Geometry: final body of the model. Coordinates: model frame, mm. Give positions to 0.01 mm unless a question says otherwise; leave off trailing zeros. Order: outer loops, then holes, each group sorted by start corner. A loop starts at its lowest first (then second) coordinate and runs counter-clockwise, first axis right, second up. Notation, with made-up numbers: (36, 10.5) - (92, 10.5) arc R30 cw to (92, 40.5) - close; hole circle Ø11 at (-19.5, 88.25). An arc over 180 degrees is marked (long way). One line per question, with ' | ' between items. Start each with the question number.
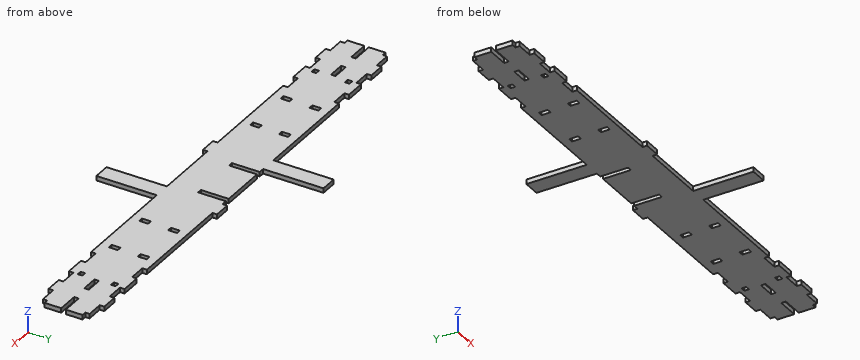
from build123d import *

# Parameters (mm, degrees)
SKETCH1_W           = 4.1
SKETCH1_H           = 4.1
SKETCH1_H_2         = 8
SKETCH1_W_2         = 15
BOSS_EXTRUDE1_DEPTH = 4.1
SKETCH2_W           = 15
SKETCH2_H           = 4.1
TOP_RIGHT_DEPTH     = 50.1
SKETCH3_W           = 15
SKETCH3_H           = 4.1
BOTTOM_LEFT_DEPTH   = 50.1


with BuildPart() as part:
    # Sketch1 → Boss-Extrude1 (new body)
    with BuildSketch(Plane.XY):
        Polygon((-205, -20.9), (-205, -25), (-190, -25), (-190, -20.9), (-175, -20.9), (-175, -25), (-157, -25), (-157, -20.9), (-142, -20.9), (-142, -25), (-45, -25), (-45, -79.2), (-30, -79.2), (-30, -25), (30, -25), (30, -79.2), (45, -79.2), (45, -25), (142, -25), (142, -20.9), (157, -20.9), (157, -25), (175, -25), (175, -20.9), (190, -20.9), (190, -25), (205, -25), (205, -20.9), (220, -20.9), (220, -17.05), (224.1, -17.05), (224.1, -2.05), (205, -2.05), (205, 2.05), (224.1, 2.05), (224.1, 17.05), (220, 17.05), (220, 20.9), (205, 20.9), (205, 25), (190, 25), (190, 20.9), (175, 20.9), (175, 25), (157, 25), (157, 20.9), (142, 20.9), (142, 25), (45, 25), (45, 79.2), (30, 79.2), (30, 25), (25, 25), (25, 0), (20.9, 0), (20.9, 25), (-20.9, 25), (-20.9, 0), (-25, 0), (-25, 25), (-30, 25), (-30, 79.2), (-45, 79.2), (-45, 25), (-142, 25), (-142, 20.9), (-157, 20.9), (-157, 25), (-175, 25), (-175, 20.9), (-190, 20.9), (-190, 25), (-205, 25), (-205, 20.9), (-220, 20.9), (-220, 17.05), (-224.1, 17.05), (-224.1, 2.05), (-205, 2.05), (-205, -2.05), (-224.1, -2.05), (-224.1, -17.05), (-220, -17.05), (-220, -20.9), align=None)
        with Locations((-172.95, -14.95)):
            Rectangle(SKETCH1_W, SKETCH1_H, mode=Mode.SUBTRACT)
        with Locations((-127.05, -13)):
            Rectangle(SKETCH1_W, SKETCH1_H_2, mode=Mode.SUBTRACT)
        with Locations((-82.05, -13)):
            Rectangle(SKETCH1_W, SKETCH1_H_2, mode=Mode.SUBTRACT)
        with Locations((82.05, -13)):
            Rectangle(SKETCH1_W, SKETCH1_H_2, mode=Mode.SUBTRACT)
        with Locations((127.05, -13)):
            Rectangle(SKETCH1_W, SKETCH1_H_2, mode=Mode.SUBTRACT)
        with Locations((172.95, -14.95)):
            Rectangle(SKETCH1_W, SKETCH1_H, mode=Mode.SUBTRACT)
        with Locations((-182.5, 0)):
            Rectangle(SKETCH1_W_2, SKETCH1_H, mode=Mode.SUBTRACT)
        with Locations((-172.95, 14.95)):
            Rectangle(SKETCH1_W, SKETCH1_H, mode=Mode.SUBTRACT)
        with Locations((-127.05, 13)):
            Rectangle(SKETCH1_W, SKETCH1_H_2, mode=Mode.SUBTRACT)
        with Locations((-82.05, 13)):
            Rectangle(SKETCH1_W, SKETCH1_H_2, mode=Mode.SUBTRACT)
        with Locations((82.05, 13)):
            Rectangle(SKETCH1_W, SKETCH1_H_2, mode=Mode.SUBTRACT)
        with Locations((127.05, 13)):
            Rectangle(SKETCH1_W, SKETCH1_H_2, mode=Mode.SUBTRACT)
        with Locations((182.5, 0)):
            Rectangle(SKETCH1_W_2, SKETCH1_H, mode=Mode.SUBTRACT)
        with Locations((172.95, 14.95)):
            Rectangle(SKETCH1_W, SKETCH1_H, mode=Mode.SUBTRACT)
    extrude(amount=BOSS_EXTRUDE1_DEPTH)

    # Sketch2 → top right (cut)
    with BuildSketch(Plane(origin=(0, 79.2, 0), x_dir=(1, 0, 0), z_dir=(0, 1, 0))):
        with Locations((37.5, -2.05)):
            Rectangle(SKETCH2_W, SKETCH2_H)
    extrude(amount=-TOP_RIGHT_DEPTH, mode=Mode.SUBTRACT)

    # Sketch3 → bottom left (cut)
    with BuildSketch(Plane.XZ.offset(79.2)):
        with Locations((-37.5, 2.05)):
            Rectangle(SKETCH3_W, SKETCH3_H)
    extrude(amount=-BOTTOM_LEFT_DEPTH, mode=Mode.SUBTRACT)


solid = part.part
(1) Cut plane C-C, the plane x = -0.5. Return the cut outline in (y, z).
(2) Contact query for flat-ended pins moving along their axis: P1, Ø2, axis at y = -22.5, z = 3, coming from the -X side; P2, Ø1.2, axis at x = -34.5, z = 1, coming from the -Y side; P3, Ø1.2, axis at x = -82.5, z = 1.5, coming from the +Y side. Output: stop coordinate, or through.
(3) Cut plane B-B, the plane y = -61.5. Return the cut outline in (x, z), plus the area to 3 significant figures.
(4) Cut plane A-A, the plane z = 2.7. Give the number of separate pieces and of enclosed holes in the cut face, plus the area to 3 significant figures.
(5) Material intervals for line 1 along Y through (x, z) = (172, 1.35); line 2 along X through (y, z) = (-0.5, 3.15); line 3 along X through (y, z) = (-22.5, 1), sorted ascending. Write a range as from..to.
Results are:
1) outline: (-25, 0) - (25, 0) - (25, 4.1) - (-25, 4.1) - close
2) P1: x = -205 | P2: y = -29.1 | P3: y = 25
3) outline: (30, 0) - (45, 0) - (45, 4.1) - (30, 4.1) - close | area: 61.5 mm2
4) separate pieces: 1 | enclosed holes: 14 | area: 22,500 mm2
5) line 1: -25..-17, -12.9..12.9, 17..25 | line 2: -205..-190, -175..175, 190..205 | line 3: -205..-190, -175..-157, -142..142, 157..175, 190..205
